Source: CAD feature listing. Evaluate the final solid. Frame: model axes, mm. Give positions to 0.01 mm unless a question says otherwise; leave off trailing zeros. Order: outer loops, then holes, each group sorted by start corner. A loop starts at its lowest first (then second) coordinate and runs counter-clockwise, first axis right, second up. Notation, with made-up numbers: M 72,-17 L 85,-17 A22 cw 85,8 Z; hole C 73,74.5 d4. An arc over 180 degrees is marked long. Answer in a Markdown table with one row per item. Add a question column.
(1) Mould query, pull axis X, two halves, no side actions, for faces 1 (the face through (-43, 67, 7)), 2 (the face through (-18, -80, 3)), 3 (the face through (-58.23, 53.39, 3.45)). Classes: pulls with the +X half, pulls with the -X half, needs draft (parallel to the pull), parting line crosses it, or undercut.
(2) Section query B-B, the plane x = 22. Return loops of the section in (y, z).
(3) Material intervals for line 1 along Z through (x, y) = (80.25, 0); line 2 along X through (y, z) = (0, 2); line 3 along X through (y, z) = (-4.5, 6.5), sorted ascending.
(4) Pin query (flat end, axial travel): P1, Ø2, axis at y = 7.5, z = 3.5, coming from the -X side; P2, Ø1.5, axis at x = 57.5, z = 3, coming from the +Y side; P3, Ø2.5, axis at y = 0, z = 3.5, coming from the +X side; P4, Ø4, axis at x = -60, z = 1.5, coming from the +Y side. Return the tip coordinate at first contact, or that it passes through.
(5) Section query A-A, the plane y = -52. Return loops of the section in (x, z).
from build123d import *

# Parameters (mm, degrees)
SKETCH1_R           = 82
SKETCH1_R_2         = 79
BOSS_EXTRUDE1_DEPTH = 7
SKETCH2_R           = 1
CUT_EXTRUDE1_DEPTH  = 125
CIRPATTERN1_COUNT   = 4


with BuildPart() as part:
    # Sketch1 → Boss-Extrude1 (new body)
    with BuildSketch(Plane.XY):
        Circle(SKETCH1_R)
        Circle(SKETCH1_R_2, mode=Mode.SUBTRACT)
    extrude(amount=BOSS_EXTRUDE1_DEPTH)

    # Sketch2 → Cut-Extrude1 (cut)
    with BuildSketch(Plane(origin=(0, 0, 0), x_dir=(1, 0, 0), z_dir=(0, 1, 0))):
        with Locations(Location((0, -3.5, 0), (0, 0, 270))):
            Circle(SKETCH2_R)
    cut_extrude1 = extrude(amount=-CUT_EXTRUDE1_DEPTH, mode=Mode.SUBTRACT)

    # CirPattern1: Cut-Extrude1 ×4 about axis
    cirpattern1_axis = Axis((0, 0, 0), (0, 0, 1))
    for i in range(1, CIRPATTERN1_COUNT):
        add(cut_extrude1.rotate(cirpattern1_axis, i * 360 / CIRPATTERN1_COUNT), mode=Mode.SUBTRACT)


solid = part.part
Values follow:
| question | item | result |
|---|---|---|
| 1 | face 1 | needs draft |
| 1 | face 2 | parting line crosses it |
| 1 | face 3 | undercut |
| 2 | outline | M -78.99,0 L -75.87,0 L -75.87,7 L -78.99,7 Z; M 75.87,0 L 78.99,0 L 78.99,7 L 75.87,7 Z |
| 3 | line 1 | z = 0 to 2.5, 4.5 to 7 |
| 3 | line 2 | x = -82 to -79, 79 to 82 |
| 3 | line 3 | x = -81.88 to -78.87, 78.87 to 81.88 |
| 4 | P1 | stops at x = -81.74 |
| 4 | P2 | stops at y = 59.19 |
| 4 | P3 | stops at x = 82 |
| 4 | P4 | stops at y = 57.97 |
| 5 | outline | M -63.4,0 L -59.47,0 L -59.47,7 L -63.4,7 Z; M 59.47,0 L 63.4,0 L 63.4,7 L 59.47,7 Z |
